Part model, mm, in its own coordinate system. Face numbers are marked on the shaded views. A direction names the side the tool comes from. Give positions to 0.01 mm unless a question says otherwise; leave off trailing zeros. Order: outer loops, then holes, each group sorted by start corner. A loop starts at its lowest first (then second) coordinate and runs counter-clockwise, first axis right, second up.
1. Slice it at D-D on z = -10. List the corners of the cut face in (x, y).
2. Drop flat-ended pins along their axis: pin 1 Ø0.8 at (x, y) = (-3, 74.5) entering from -Z (3 decimals); pin 2 Ø1.5 at (x, y) = (-3, 73.5) entering from +Z. Give the stop position or say it passes through.
3. Slice it at C-C on y = 79.25. List the corners of the cut face in (x, z) (3 decimals).
4. Slice it at A-A on x = -3.5. List the corners of the cut face in (y, z) (3 decimals).
5. Probe line 1 (Z direction, x = -3, y = 80) (3 decimals); line 2 (Y direction, x = -2.8, z = 3); line 3 (Y direction, x = -3.4, z = -14.5). List the from-to ranges inside material, lowest first.
6. Slice it at B-B on z = 4.5. List the corners of the cut face in (x, y).
7. Which spindle directions (+Z, -Z, +X, -X, +Y, -Y) get a long thin tool onto all of the face, cutting with end or side? Do the marked faces 1 and 2. Say none if no direction does.
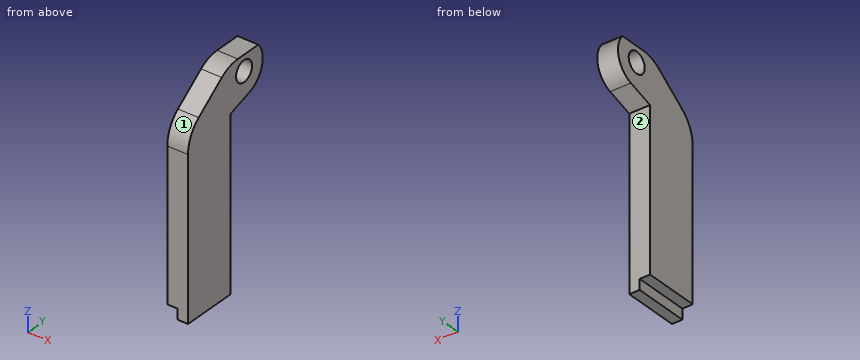
from build123d import *

# Parameters (mm, degrees)
TAB_EXTRUDE_DEPTH       = 8
SKETCH3_R               = 1.5
SCREWHOLE_EXTRUDE_DEPTH = 3
STRUCTURAL_ROUNDING_R   = 5


with BuildPart() as part:
    # Sketch1 → Tab extrude (new body)
    with BuildSketch(Plane.XZ.offset(-69.5)):
        Polygon((-1, 0.185), (-1, -25.315), (-2.5, -25.315), (-2.5, -23.815), (-4, -23.815), (-4, 0.185), align=None)
    extrude(amount=-TAB_EXTRUDE_DEPTH)

    # Sketch3 → Screwhole extrude (add)
    with BuildSketch(Plane.ZY.offset(1)):
        with BuildLine():
            Line((0.185, 69.5), (5.935, 77.166666667))
            Line((5.935, 77.166666667), (5.935, 82.680951324))
            ThreePointArc((5.935, 82.680951324), (2.723639085, 83.365380393), (0.35837639, 81.087922497))
            Line((0.35837639, 81.087922497), (-0.815, 77.5))
            Line((-0.815, 77.5), (0.185, 77.5))
            Line((0.185, 77.5), (0.185, 69.5))
        make_face()
        with Locations((3.685, 80)):
            Circle(SKETCH3_R, mode=Mode.SUBTRACT)
    extrude(amount=SCREWHOLE_EXTRUDE_DEPTH)

    # Structural rounding
    structural_rounding_edges = [part.edges().sort_by_distance(p)[0] for p in [
        (-2.5, 77.166666667, 5.935),
        (-2.5, 69.5, 0.185),
    ]]
    fillet(structural_rounding_edges, radius=STRUCTURAL_ROUNDING_R)


solid = part.part
Data:
1. outline: (-4, 69.5) - (-1, 69.5) - (-1, 77.5) - (-4, 77.5) - close
2. pin 1: stops at z = -23.815
2. pin 2: stops at z = 3.75
3. outline: (-4, -0.243) - (-1, -0.243) - (-1, 2.386) - (-4, 2.386) - close; (-4, 4.984) - (-1, 4.984) - (-1, 5.935) - (-4, 5.935) - close
4. outline: (69.5, -23.815) - (77.5, -23.815) - (77.5, -0.815) - (81.088, 0.358) arc R3.5 ccw to (82.681, 5.935) - (78.833, 5.935) arc R5 ccw to (75.833, 4.935) - (71.5, 1.685) arc R5 ccw to (69.5, -2.315) - close; hole circle Ø3 at (80, 3.685)
5. line 1: z = 0.003 to 2.185, 5.185 to 5.935
5. line 2: y = 73.25 to 78.67, 81.33 to 83.43
5. line 3: y = 69.5 to 77.5
6. outline: (-4, 75.25) - (-1, 75.25) - (-1, 78.74) - (-4, 78.74) - close; (-4, 81.26) - (-1, 81.26) - (-1, 83.4) - (-4, 83.4) - close
7. face 1: +Z, +X, -X, -Y
7. face 2: -Z, +X, -X, +Y
